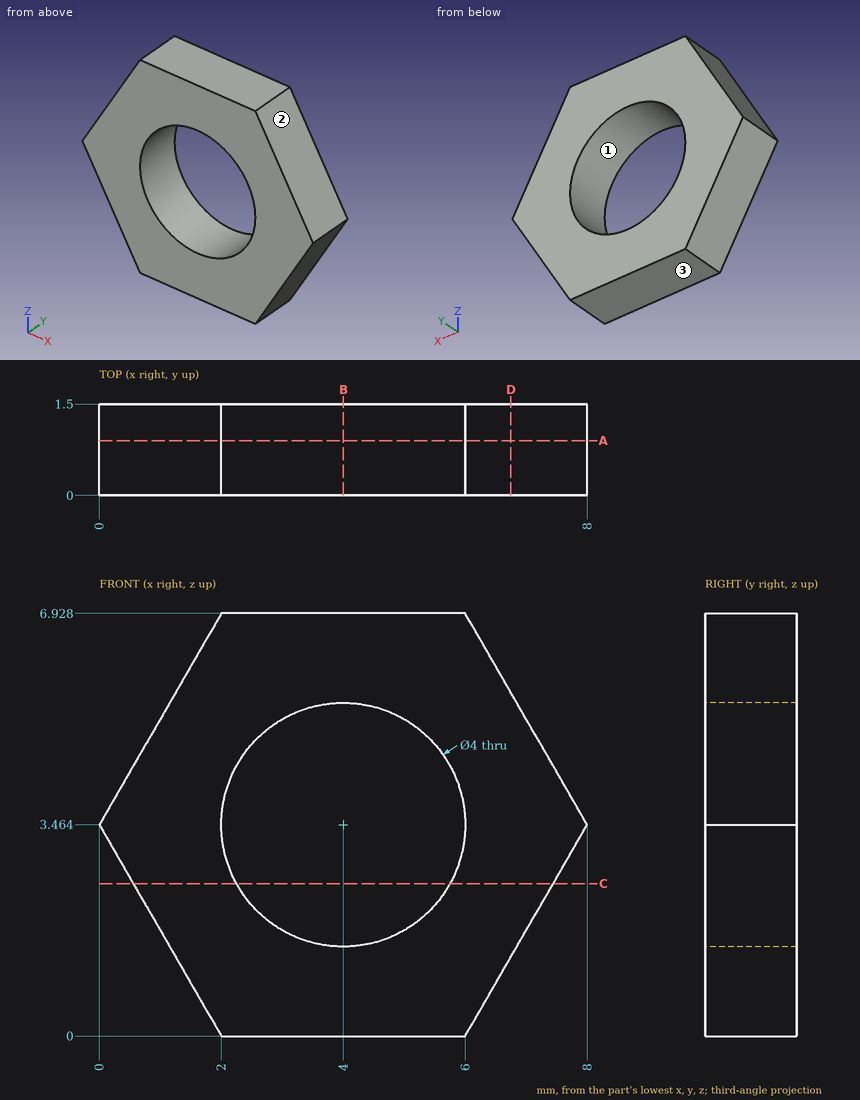
Check sheet for the drawn part. Datum: minimum x, y, z corner. Units: mm. Round coordinates to 2 decimals unless told otherwise and drop trailing zeros. Write each loop counter-clockwise with the first axis right and the second up, starting at its lowest first coordinate (ties: lowest second). Pieces come first, ordered by that corner, then holes. Notation, with made-up numbers: (13.5, 61.25) -> (37.5, 61.25) arc R11 ccw to (37.5, 72.25) -> close; hole circle Ø11 at (0.25, -34.5). An arc over 180 degrees is marked (long way). One line per item, written item: value. Start each with the question number.
(1) Cross-section at D-D, the plane x = 6.75. Record the cut outline in (y, z).
(2) Cross-section at C-C, the plane z = 2.5. Record the cut outline in (x, y).
(3) Cross-section at A-A, the plane y = 0.9. Record the cut outline in (x, z).
(4) Draft check along X on the marked faces 1, 2 and 3. Enter one of: +X half, -X half, draft (parallel to the pull), parting line (faces both ways), or undercut.
(5) Cross-section at B-B, the plane x = 4. Record the cut outline in (y, z).
(6) Scan lines: line 1 (Z direction, x = 4, y = 0.8); line 2 (Z direction, x = 2.25, y = 1.3) (1 decimal); line 3 (X direction, y = 1.1, z = 1.75). Record each from-to range of solid material in increasing order. Write a range as [from, to].
Answer:
1. outline: (0, 1.3) -> (1.5, 1.3) -> (1.5, 5.63) -> (0, 5.63) -> close
2. outline: (0.56, 0) -> (2.25, 0) -> (2.25, 1.5) -> (0.56, 1.5) -> close; (5.75, 0) -> (7.44, 0) -> (7.44, 1.5) -> (5.75, 1.5) -> close
3. outline: (0, 3.46) -> (2, 0) -> (6, 0) -> (8, 3.46) -> (6, 6.93) -> (2, 6.93) -> close; hole circle Ø4 at (4, 3.46)
4. face 1: undercut
4. face 2: +X half
4. face 3: draft
5. outline: (0, 0) -> (1.5, 0) -> (1.5, 1.46) -> (0, 1.46) -> close; (0, 5.46) -> (1.5, 5.46) -> (1.5, 6.93) -> (0, 6.93) -> close
6. line 1: [0, 1.46], [5.46, 6.93]
6. line 2: [0, 2.5], [4.4, 6.9]
6. line 3: [0.99, 2.97], [5.03, 7.01]
